from build123d import *

# Parameters (mm, degrees)
EXTRUDE_1_DEPTH   = 2
HOLE_WIZARD_M81_D = 9
CHAMFER_1_SIZE    = 2


with BuildPart() as part:
    # Эскиз1 → Бобышка-Вытянуть1 (new body)
    with BuildSketch(Plane(origin=(0, 0, 0), x_dir=(1, 0, 0), z_dir=(0, 0, -1))):
        Polygon((0, 0), (0, 80), (80, 80), (80, 40), (40, 0), align=None)
    extrude(amount=EXTRUDE_1_DEPTH)

    # Отверстие с зазором M81 (through all)
    with Locations(Plane(origin=(0, 0, -2), x_dir=(1, 0, 0), z_dir=(0, 0, -1))):
        with Locations((20, 60), (20, 20), (60, 60)):
            Hole(HOLE_WIZARD_M81_D / 2)

    # Фаска1
    chamfer_1_edges = [part.edges().sort_by_distance(p)[0] for p in [
        (0, 0, -1),
        (0, -80, -1),
        (80, -80, -1),
    ]]
    chamfer(chamfer_1_edges, length=CHAMFER_1_SIZE)


solid = part.part
Work out the finished part from the listing and answer in its coordinate system (mm). Give positions to 0.01 mm unless a question says otherwise; leave off trailing zeros. Write each loop counter-clockwise with the first axis right and the second up, starting at its lowest first coordinate (ties: lowest second). Pieces come first, ordered by that corner, then holes.
Q1. The part is cut by section D-D on x = 20. Give the vertices of the cut face in (y, z), and give its area (3 significant figures).
Answer:
outline: (-80, -2) - (-64.5, -2) - (-64.5, 0) - (-80, 0) - close; (-55.5, -2) - (-24.5, -2) - (-24.5, 0) - (-55.5, 0) - close; (-15.5, -2) - (0, -2) - (0, 0) - (-15.5, 0) - close
area: 124 mm2
Q2. For a pull along X with two mould halves and no side action, classify faces 1 (the face through (1, -1, -1)), 2 (the face through (60, -20, -1)), 3 (the face through (41, -41, -2)), 4 (the face through (23.32, -23.04, -0.99)) as released by +X, released by -X, zero draft, split by the parting line, or undercut.
Answer:
face 1: released by -X
face 2: released by +X
face 3: zero draft
face 4: undercut
Q3. The part is cut by section B-B on y = -60. Give the vertices of the cut face in (x, z), and give its area (3 significant figures).
Answer:
outline: (0, -2) - (15.5, -2) - (15.5, 0) - (0, 0) - close; (24.5, -2) - (55.5, -2) - (55.5, 0) - (24.5, 0) - close; (64.5, -2) - (80, -2) - (80, 0) - (64.5, 0) - close
area: 124 mm2
Q4. The part is cut by section A-A on x = 60. Give the vertices of the cut face in (y, z), and give its area (3 significant figures).
Answer:
outline: (-80, -2) - (-64.5, -2) - (-64.5, 0) - (-80, 0) - close; (-55.5, -2) - (-20, -2) - (-20, 0) - (-55.5, 0) - close
area: 102 mm2
Q5. Given pin 1 (12 mm diameter, centred on x = 64, y = -15, fed in from -Z); pin 2 (1 mm diameter, centred on x = 70.5, z = -1.5, fed in from +Y), each flat-ended and moving along its own axis, determine where each tip first touches the part or whether it passes through.
Answer:
pin 1: passes through
pin 2: stops at y = -30
Q6. The part is cut by section C-C on z = -0.45. Give the vertices of the cut face in (x, y).
Answer:
outline: (0, -78) - (2, -80) - (78, -80) - (80, -78) - (80, -40) - (40, 0) - (2, 0) - (0, -2) - close; hole circle Ø9 at (20, -60); hole circle Ø9 at (20, -20); hole circle Ø9 at (60, -60)
Q7. Straight lines are drawn through the part: L1, parallel to X at y = -60, z = -0.8; L2, parallel to Y at x = 20, z = -1.6; L3, parallel to Y at x = 18.5, z = -0.25. For each, find the intervals that lie inside material, in ascending order.
Answer:
L1: x = 0 to 15.5, 24.5 to 55.5, 64.5 to 80
L2: y = -80 to -64.5, -55.5 to -24.5, -15.5 to 0
L3: y = -80 to -64.24, -55.76 to -24.24, -15.76 to 0
